Design review of the part built by this model. Coordinates are the model's own, in mm. A direction names the side the tool comes from. Give positions to 0.01 mm unless a question says otherwise; leave off trailing zeros. Write each loop counter-clockwise with the first axis right and the second up, starting at its lowest first coordinate (ties: lowest second). Pieces come first, ordered by that corner, then holes. Notation, with made-up numbers: M -1.75,87 L 2.25,87 A10 cw 2.25,104 Z; hole C 58.25,-29.5 d4. An arc over 180 degrees is marked long. Answer in a Markdown table with one row per item.
```python
from build123d import *

# Parameters (mm, degrees)
SKETCH2_W           = 50
SKETCH2_H           = 50
BOSS_EXTRUDE2_DEPTH = 14
SKETCH4_R           = 2.75
CUT_EXTRUDE1_DEPTH  = 12
BOSS_EXTRUDE3_DEPTH = 20
SKETCH8_W           = 50
SKETCH8_H           = 50
BOSS_EXTRUDE4_DEPTH = 8
CUT_EXTRUDE3_REACH  = 56.9
CUT_EXTRUDE4_REACH  = 56.9
SKETCH10_R          = 10


with BuildPart() as part:
    # Sketch2 → Boss-Extrude2 (new body)
    with BuildSketch(Plane.XY):
        Rectangle(SKETCH2_W, SKETCH2_H)
    extrude(amount=BOSS_EXTRUDE2_DEPTH)

    # Sketch4 → Cut-Extrude1 (cut)
    with BuildSketch(Plane(origin=(0, 0, 0), x_dir=(-1, 0, 0), z_dir=(0, 0, -1))):
        with Locations((-16.5, 16.5)):
            Circle(SKETCH4_R)
        with Locations((16.5, 16.5)):
            Circle(SKETCH4_R)
        with Locations((16.5, -16.5)):
            Circle(SKETCH4_R)
        with Locations((-16.5, -16.5)):
            Circle(SKETCH4_R)
    extrude(amount=-CUT_EXTRUDE1_DEPTH, mode=Mode.SUBTRACT)

    # Sketch5 → Boss-Extrude3 (add)
    with BuildSketch(Plane.XY.offset(14)):
        Polygon((25, 15.5), (11.143593539, 7.5), (7.5, 11.143593539), (15.5, 25), (-15.5, 25), (-7.5, 11.143593539), (-11.143593539, 7.5), (-25, 15.5), (-25, -15.5), (-11.143593539, -7.5), (-7.5, -11.143593539), (-15.5, -25), (15.5, -25), (7.5, -11.143593539), (11.143593539, -7.5), (25, -15.5), align=None)
    extrude(amount=BOSS_EXTRUDE3_DEPTH)

    # Sketch8 → Boss-Extrude4 (add)
    with BuildSketch(Plane.XY.offset(34)):
        Rectangle(SKETCH8_W, SKETCH8_H)
    extrude(amount=BOSS_EXTRUDE4_DEPTH)

    # Sketch9 → Cut-Extrude3 (cut, up to next)
    with BuildSketch(Plane.XY.offset(42), mode=Mode.PRIVATE) as cut_extrude3_sk1:
        with BuildLine():
            ThreePointArc((14.5, 12), (12, 14.5), (9.5, 12))
            Line((9.5, 12), (12, 12))
            Line((12, 12), (12, 9.5))
            ThreePointArc((12, 9.5), (13.767766953, 10.232233047), (14.5, 12))
        make_face()
    cut_extrude3_tool1 = extrude(cut_extrude3_sk1.sketch, amount=-CUT_EXTRUDE3_REACH, mode=Mode.PRIVATE) & part.part
    # Sketch9 → Cut-Extrude3 (cut, up to next)
    with BuildSketch(Plane.XY.offset(42), mode=Mode.PRIVATE) as cut_extrude3_sk2:
        with BuildLine():
            Line((12, 12), (9.5, 12))
            ThreePointArc((9.5, 12), (10.232233047, 10.232233047), (12, 9.5))
            Line((12, 9.5), (12, 12))
        make_face()
    cut_extrude3_tool2 = extrude(cut_extrude3_sk2.sketch, amount=-CUT_EXTRUDE3_REACH, mode=Mode.PRIVATE) & part.part
    # Sketch9 → Cut-Extrude3 (cut, up to next)
    with BuildSketch(Plane.XY.offset(42), mode=Mode.PRIVATE) as cut_extrude3_sk3:
        with BuildLine():
            ThreePointArc((14.5, 12), (12, 14.5), (9.5, 12))
            Line((9.5, 12), (12, 12))
            Line((12, 12), (12, 9.5))
            ThreePointArc((12, 9.5), (13.767766953, 10.232233047), (14.5, 12))
        make_face()
    cut_extrude3_tool3 = extrude(cut_extrude3_sk3.sketch, amount=-CUT_EXTRUDE3_REACH, mode=Mode.PRIVATE) & part.part
    # Sketch9 → Cut-Extrude3 (cut, up to next)
    with BuildSketch(Plane.XY.offset(42), mode=Mode.PRIVATE) as cut_extrude3_sk4:
        with BuildLine():
            Line((12, 12), (9.5, 12))
            ThreePointArc((9.5, 12), (10.232233047, 10.232233047), (12, 9.5))
            Line((12, 9.5), (12, 12))
        make_face()
    cut_extrude3_tool4 = extrude(cut_extrude3_sk4.sketch, amount=-CUT_EXTRUDE3_REACH, mode=Mode.PRIVATE) & part.part
    # Sketch9 → Cut-Extrude3 (cut, up to next)
    with BuildSketch(Plane.XY.offset(42), mode=Mode.PRIVATE) as cut_extrude3_sk5:
        with BuildLine():
            ThreePointArc((14.5, -12), (13.767766953, -10.232233047), (12, -9.5))
            Line((12, -9.5), (12, -12))
            Line((12, -12), (9.5, -12))
            ThreePointArc((9.5, -12), (12, -14.5), (14.5, -12))
        make_face()
    cut_extrude3_tool5 = extrude(cut_extrude3_sk5.sketch, amount=-CUT_EXTRUDE3_REACH, mode=Mode.PRIVATE) & part.part
    # Sketch9 → Cut-Extrude3 (cut, up to next)
    with BuildSketch(Plane.XY.offset(42), mode=Mode.PRIVATE) as cut_extrude3_sk6:
        with BuildLine():
            Line((12, -12), (12, -9.5))
            ThreePointArc((12, -9.5), (10.232233047, -10.232233047), (9.5, -12))
            Line((9.5, -12), (12, -12))
        make_face()
    cut_extrude3_tool6 = extrude(cut_extrude3_sk6.sketch, amount=-CUT_EXTRUDE3_REACH, mode=Mode.PRIVATE) & part.part
    # Sketch9 → Cut-Extrude3 (cut, up to next)
    with BuildSketch(Plane.XY.offset(42), mode=Mode.PRIVATE) as cut_extrude3_sk7:
        with BuildLine():
            ThreePointArc((14.5, -12), (13.767766953, -10.232233047), (12, -9.5))
            Line((12, -9.5), (12, -12))
            Line((12, -12), (9.5, -12))
            ThreePointArc((9.5, -12), (12, -14.5), (14.5, -12))
        make_face()
    cut_extrude3_tool7 = extrude(cut_extrude3_sk7.sketch, amount=-CUT_EXTRUDE3_REACH, mode=Mode.PRIVATE) & part.part
    # Sketch9 → Cut-Extrude3 (cut, up to next)
    with BuildSketch(Plane.XY.offset(42), mode=Mode.PRIVATE) as cut_extrude3_sk8:
        with BuildLine():
            Line((12, -12), (12, -9.5))
            ThreePointArc((12, -9.5), (10.232233047, -10.232233047), (9.5, -12))
            Line((9.5, -12), (12, -12))
        make_face()
    cut_extrude3_tool8 = extrude(cut_extrude3_sk8.sketch, amount=-CUT_EXTRUDE3_REACH, mode=Mode.PRIVATE) & part.part
    # Sketch9 → Cut-Extrude3 (cut, up to next)
    with BuildSketch(Plane.XY.offset(42), mode=Mode.PRIVATE) as cut_extrude3_sk9:
        with BuildLine():
            ThreePointArc((-9.5, -12), (-10.232233047, -10.232233047), (-12, -9.5))
            Line((-12, -9.5), (-12, -12))
            Line((-12, -12), (-9.5, -12))
        make_face()
    cut_extrude3_tool9 = extrude(cut_extrude3_sk9.sketch, amount=-CUT_EXTRUDE3_REACH, mode=Mode.PRIVATE) & part.part
    # Sketch9 → Cut-Extrude3 (cut, up to next)
    with BuildSketch(Plane.XY.offset(42), mode=Mode.PRIVATE) as cut_extrude3_sk10:
        with BuildLine():
            Line((-12, -12), (-12, -9.5))
            ThreePointArc((-12, -9.5), (-13.767766953, -13.767766953), (-9.5, -12))
            Line((-9.5, -12), (-12, -12))
        make_face()
    cut_extrude3_tool10 = extrude(cut_extrude3_sk10.sketch, amount=-CUT_EXTRUDE3_REACH, mode=Mode.PRIVATE) & part.part
    # Sketch9 → Cut-Extrude3 (cut, up to next)
    with BuildSketch(Plane.XY.offset(42), mode=Mode.PRIVATE) as cut_extrude3_sk11:
        with BuildLine():
            ThreePointArc((-9.5, -12), (-10.232233047, -10.232233047), (-12, -9.5))
            Line((-12, -9.5), (-12, -12))
            Line((-12, -12), (-9.5, -12))
        make_face()
    cut_extrude3_tool11 = extrude(cut_extrude3_sk11.sketch, amount=-CUT_EXTRUDE3_REACH, mode=Mode.PRIVATE) & part.part
    # Sketch9 → Cut-Extrude3 (cut, up to next)
    with BuildSketch(Plane.XY.offset(42), mode=Mode.PRIVATE) as cut_extrude3_sk12:
        with BuildLine():
            Line((-12, -12), (-12, -9.5))
            ThreePointArc((-12, -9.5), (-13.767766953, -13.767766953), (-9.5, -12))
            Line((-9.5, -12), (-12, -12))
        make_face()
    cut_extrude3_tool12 = extrude(cut_extrude3_sk12.sketch, amount=-CUT_EXTRUDE3_REACH, mode=Mode.PRIVATE) & part.part
    # Sketch9 → Cut-Extrude3 (cut, up to next)
    with BuildSketch(Plane.XY.offset(42), mode=Mode.PRIVATE) as cut_extrude3_sk13:
        with BuildLine():
            Line((-12, 9.5), (-12, 12))
            Line((-12, 12), (-9.5, 12))
            ThreePointArc((-9.5, 12), (-13.767766953, 13.767766953), (-12, 9.5))
        make_face()
    cut_extrude3_tool13 = extrude(cut_extrude3_sk13.sketch, amount=-CUT_EXTRUDE3_REACH, mode=Mode.PRIVATE) & part.part
    # Sketch9 → Cut-Extrude3 (cut, up to next)
    with BuildSketch(Plane.XY.offset(42), mode=Mode.PRIVATE) as cut_extrude3_sk14:
        with BuildLine():
            Line((-9.5, 12), (-12, 12))
            Line((-12, 12), (-12, 9.5))
            ThreePointArc((-12, 9.5), (-10.232233047, 10.232233047), (-9.5, 12))
        make_face()
    cut_extrude3_tool14 = extrude(cut_extrude3_sk14.sketch, amount=-CUT_EXTRUDE3_REACH, mode=Mode.PRIVATE) & part.part
    # Sketch9 → Cut-Extrude3 (cut, up to next)
    with BuildSketch(Plane.XY.offset(42), mode=Mode.PRIVATE) as cut_extrude3_sk15:
        with BuildLine():
            Line((-12, 9.5), (-12, 12))
            Line((-12, 12), (-9.5, 12))
            ThreePointArc((-9.5, 12), (-13.767766953, 13.767766953), (-12, 9.5))
        make_face()
    cut_extrude3_tool15 = extrude(cut_extrude3_sk15.sketch, amount=-CUT_EXTRUDE3_REACH, mode=Mode.PRIVATE) & part.part
    # Sketch9 → Cut-Extrude3 (cut, up to next)
    with BuildSketch(Plane.XY.offset(42), mode=Mode.PRIVATE) as cut_extrude3_sk16:
        with BuildLine():
            Line((-9.5, 12), (-12, 12))
            Line((-12, 12), (-12, 9.5))
            ThreePointArc((-12, 9.5), (-10.232233047, 10.232233047), (-9.5, 12))
        make_face()
    cut_extrude3_tool16 = extrude(cut_extrude3_sk16.sketch, amount=-CUT_EXTRUDE3_REACH, mode=Mode.PRIVATE) & part.part
    add(cut_extrude3_tool1.solids().sort_by_distance((12.353678, 12.353678, 42))[0], mode=Mode.SUBTRACT)
    add(cut_extrude3_tool2.solids().sort_by_distance((10.938967, 10.938967, 42))[0], mode=Mode.SUBTRACT)
    add(cut_extrude3_tool3.solids().sort_by_distance((12.353678, 12.353678, 42))[0], mode=Mode.SUBTRACT)
    add(cut_extrude3_tool4.solids().sort_by_distance((10.938967, 10.938967, 42))[0], mode=Mode.SUBTRACT)
    add(cut_extrude3_tool5.solids().sort_by_distance((12.353678, -12.353678, 42))[0], mode=Mode.SUBTRACT)
    add(cut_extrude3_tool6.solids().sort_by_distance((10.938967, -10.938967, 42))[0], mode=Mode.SUBTRACT)
    add(cut_extrude3_tool7.solids().sort_by_distance((12.353678, -12.353678, 42))[0], mode=Mode.SUBTRACT)
    add(cut_extrude3_tool8.solids().sort_by_distance((10.938967, -10.938967, 42))[0], mode=Mode.SUBTRACT)
    add(cut_extrude3_tool9.solids().sort_by_distance((-10.938967, -10.938967, 42))[0], mode=Mode.SUBTRACT)
    add(cut_extrude3_tool10.solids().sort_by_distance((-12.353678, -12.353678, 42))[0], mode=Mode.SUBTRACT)
    add(cut_extrude3_tool11.solids().sort_by_distance((-10.938967, -10.938967, 42))[0], mode=Mode.SUBTRACT)
    add(cut_extrude3_tool12.solids().sort_by_distance((-12.353678, -12.353678, 42))[0], mode=Mode.SUBTRACT)
    add(cut_extrude3_tool13.solids().sort_by_distance((-12.353678, 12.353678, 42))[0], mode=Mode.SUBTRACT)
    add(cut_extrude3_tool14.solids().sort_by_distance((-10.938967, 10.938967, 42))[0], mode=Mode.SUBTRACT)
    add(cut_extrude3_tool15.solids().sort_by_distance((-12.353678, 12.353678, 42))[0], mode=Mode.SUBTRACT)
    add(cut_extrude3_tool16.solids().sort_by_distance((-10.938967, 10.938967, 42))[0], mode=Mode.SUBTRACT)

    # Sketch10 → Cut-Extrude4 (cut, up to next)
    with BuildSketch(Plane.XY.offset(42), mode=Mode.PRIVATE) as cut_extrude4_sk1:
        Circle(SKETCH10_R)
    cut_extrude4_tool1 = extrude(cut_extrude4_sk1.sketch, amount=-CUT_EXTRUDE4_REACH, mode=Mode.PRIVATE) & part.part
    add(cut_extrude4_tool1.solids().sort_by_distance((0, 0, 42))[0], mode=Mode.SUBTRACT)


solid = part.part
```
1) Insertion check: P1, Ø1.6, axis at x = 16, y = -16, coming from the -Z side; P2, Ø10, axis at x = 1, y = 6, coming from the -Z side. Each pin has a flat end and moves straight along its axis. Give the tip position at first contact, or say it passes through.
Geometry says:
| item | result |
|---|---|
| P1 | z = 12 |
| P2 | z = 0 |
2) Add section A-A (z = 38). Write out the cut boundary in (x, y), and give its area (3 significant figures).
Geometry says:
| item | result |
|---|---|
| outline | M -25,-25 L 25,-25 L 25,25 L -25,25 Z; hole C -12,-12 d5; hole C -12,12 d5; hole C 0,0 d20; hole C 12,-12 d5; hole C 12,12 d5 |
| area | 2,110 mm^2 |
3) Add section D-D (y = 8.5). Write out the cut boundary in (x, z).
Geometry says:
| item | result |
|---|---|
| outline | M -25,0 L -5.27,0 L -5.27,42 L -25,42 Z; M 5.27,0 L 25,0 L 25,42 L 5.27,42 Z; hole M -12.88,14 L -10.14,14 L -10.14,34 L -12.88,34 Z; hole M 10.14,14 L 12.88,14 L 12.88,34 L 10.14,34 Z |
4) For faces 1 (the face through (17, -16, 12)), 2 (the face through (0, -25, 21)), 3 (the face through (16, -16, 14)), list the 3-axis set-ups (+Z, -Z, +X, -X, +Y, -Y) from which the entire face can be reached by the end or side of a thin tool; tool diameter is ignored.
Geometry says:
| item | result |
|---|---|
| face 1 | -Z |
| face 2 | +Z, -Z, +X, -X, -Y |
| face 3 | none |
5) To check wall thickness, follow probe 1 along Y at (x, z) = (-16.5, 8.5); probe 2 along Y at (x, z) = (-12, 39); probe 3 along Z at (x, y) = (-18.5, 22). State the ranges of each line that lie inside material, in increasing order. Write a range as [from, to].
Geometry says:
| item | result |
|---|---|
| probe 1 | [-25, -19.25], [-13.75, 13.75], [19.25, 25] |
| probe 2 | [-25, -14.5], [-9.5, 9.5], [14.5, 25] |
| probe 3 | [0, 14], [34, 42] |
6) Add section B-B (y = 0). Write out the cut boundary in (x, z).
Geometry says:
| item | result |
|---|---|
| outline | M -25,0 L -10,0 L -10,42 L -25,42 Z; M 10,0 L 25,0 L 25,42 L 10,42 Z |
7) The part is to be moulded in two halves that separate along Z. For faces 4 (the face through (17, 17, 12)), 5 (the face through (25, 0, 21)), 6 (the face through (-11.44, -17.97, 23.86)), 7 (the face through (17.97, -11.44, 23.86)), say which applies: released by +Z, released by -Z, zero draft, split by the parting line, or undercut.
Geometry says:
| item | result |
|---|---|
| face 4 | released by -Z |
| face 5 | zero draft |
| face 6 | undercut |
| face 7 | undercut |
